The drawing under review shows one solid part. Ordinate dimensions are in mm from its lowest x, y, z. A direction names the side the tool comes from. Give positions to 0.01 mm unless a question says otherwise; leave off trailing zeros. Write each loop counter-clockwise with the first axis right and the second up, starting at its lowest first coordinate (ties: lowest second). Pieces come first, ordered by that corner, then holes. Notation, with made-up numbers: M 45.25,67.5 L 54.25,67.5 A16 cw 54.25,83.5 Z; hole C 73,86 d6. An arc over 180 degrees is marked long. One line per item, written item: value. Start each with the question number.
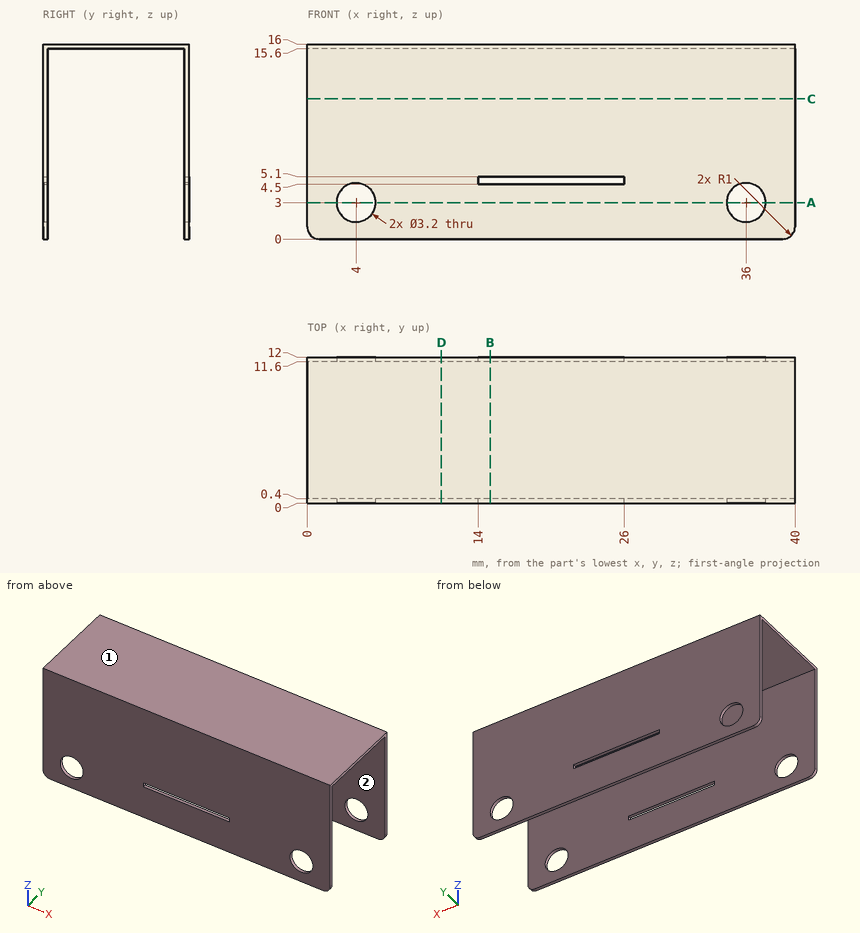
Q1. Take a section at C-C, the plane z = 11.5. Give the boundary of the cut face in (x, y).
Q2. Wall thickness on line 1 (Y direction, x = 11, z = 5); line 2 (Z direction, x = 4, y = 0.3); line 3 (Z direction, x = 34, y = 8): over which ranges is each line inside the solid? List them lowest first. Write a range as from..to.
Q3. Take a section at A-A, the plane z = 3. Give the boundary of the cut face in (x, y).
Q4. Take a section at B-B, the plane x = 15. Give the boundary of the cut face in (y, z), then the cut area to 3 significant figures.
Q5. Take a section at D-D, the plane x = 11. Give the boundary of the cut face in (y, z).
Q6. For P1, Ø4, axis at y = 8.5, z = 5, coming from the -X side; P2, Ø3.5, axis at x = 12.5, y = 4.5, coming from the -Z side, all flat-tipped, find the tip position at first contact; note any pin that passes through.
Q7. Machinability: for the marked faces 1 and 2, which of the approach directions +Z, -Z, +X, -X, +Y, -Y give a long, thin tool a straight path to every point of the face, cutting with its end or side? Answer none if there is none.
Results list:
1. outline: M 0,0 L 40,0 L 40,0.4 L 0,0.4 Z; M 0,11.6 L 40,11.6 L 40,12 L 0,12 Z
2. line 1: y = 0..0.4, 11.6..12
2. line 2: z = 0..1.4, 4.6..16
2. line 3: z = 15.6..16
3. outline: M 0,0 L 2.4,0 L 2.4,0.4 L 0,0.4 Z; M 0,11.6 L 2.4,11.6 L 2.4,12 L 0,12 Z; M 5.6,0 L 34.4,0 L 34.4,0.4 L 5.6,0.4 Z; M 5.6,11.6 L 34.4,11.6 L 34.4,12 L 5.6,12 Z; M 37.6,0 L 40,0 L 40,0.4 L 37.6,0.4 Z; M 37.6,11.6 L 40,11.6 L 40,12 L 37.6,12 Z
4. outline: M 0,0 L 0.4,0 L 0.4,4.5 L 0,4.5 Z; M 0,5.1 L 0.4,5.1 L 0.4,15.6 L 11.6,15.6 L 11.6,5.1 L 12,5.1 L 12,16 L 0,16 Z; M 11.6,0 L 12,0 L 12,4.5 L 11.6,4.5 Z
4. area: 16.8 mm^2
5. outline: M 0,0 L 0.4,0 L 0.4,15.6 L 11.6,15.6 L 11.6,0 L 12,0 L 12,16 L 0,16 Z
6. P1: passes through
6. P2: stops at z = 15.6
7. face 1: +Z, +X, -X, +Y, -Y
7. face 2: -Z, +X, -X
